Here's how the part is built. I have some questions about the finished solid (model axes, mm). Face numbers are marked on the shaded views. Round coordinates to 2 decimals unless told otherwise and drop trailing zeros. Loops run counter-clockwise (first coordinate to the right, second up) from the corner with the lowest first, then second, coordinate; pieces in that order, holes last. Notation, with made-up numbers: M 10.5,66 L 29.5,66 A26 ccw 29.5,87 Z; hole C 13.5,70.25 d8. An arc over 180 degrees is marked long. Use a Markdown table: item, result.
from build123d import *

# Parameters (mm, degrees)
SKETCH_1_W                   = 20
SKETCH_1_H                   = 50
SKETCH_1_R                   = 3.3
SCREW_BRACKET_20X50X40_DEPTH = 40
SKETCH_2_R                   = 4.25
M10_TAP_PILOT_8P5_DEPTH      = 20


with BuildPart() as part:
    # 草图1 → Screw_bracket_20x50x40 (new body)
    with BuildSketch(Plane.XY):
        with Locations((10, 25)):
            Rectangle(SKETCH_1_W, SKETCH_1_H)
        with Locations((10, 8)):
            Circle(SKETCH_1_R, mode=Mode.SUBTRACT)
        with Locations((10, 42)):
            Circle(SKETCH_1_R, mode=Mode.SUBTRACT)
    extrude(amount=SCREW_BRACKET_20X50X40_DEPTH)

    # 草图2 → M10_tap_pilot_8p5 (cut)
    with BuildSketch(Plane.ZY):
        with Locations((20, 25)):
            Circle(SKETCH_2_R)
    extrude(amount=-M10_TAP_PILOT_8P5_DEPTH, mode=Mode.SUBTRACT)


solid = part.part
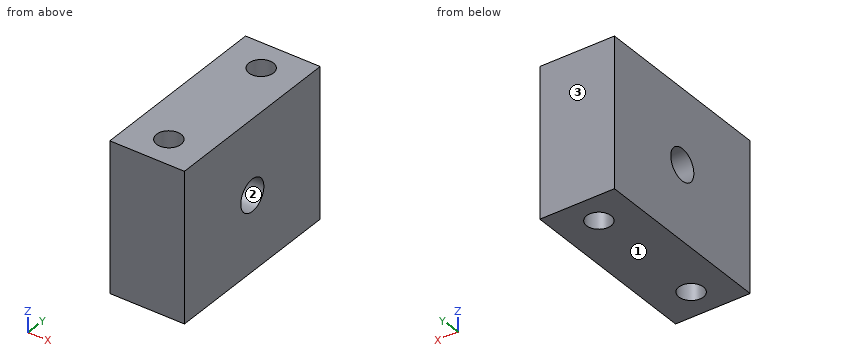
1. Imagine slicing it at D-D, the plane z = 9.5. Write out the boundary of the cut face in (x, y), then the cut area to 3 significant figures.
Answer sheet:
| item | result |
|---|---|
| outline | M 0,0 L 20,0 L 20,50 L 0,50 Z; hole C 10,8 d6.6; hole C 10,42 d6.6 |
| area | 932 mm2 |
2. Imagine slicing it at A-A, the plane z = 18. Write out the boundary of the cut face in (x, y).
Answer sheet:
| item | result |
|---|---|
| outline | M 0,0 L 20,0 L 20,21.25 L 0,21.25 Z; M 0,28.75 L 20,28.75 L 20,50 L 0,50 Z; hole C 10,8 d6.6; hole C 10,42 d6.6 |
3. I need wall thicknesses on probe 1 along Y at (x, z) = (10, 10); probe 2 along Y at (x, z) = (8, 17); probe 3 along Y at (x, z) = (10, 17). Which ranges of each line are inside material? Lowest first, please. Write a range as from..to.
Answer sheet:
| item | result |
|---|---|
| probe 1 | 0..4.7, 11.3..38.7, 45.3..50 |
| probe 2 | 0..5.38, 10.62..21.99, 28.01..39.38, 44.62..50 |
| probe 3 | 0..4.7, 11.3..21.99, 28.01..38.7, 45.3..50 |
4. Imagine slicing it at C-C, the plane y = 42. Write out the boundary of the cut face in (x, z), then the cut area to 3 significant figures.
Answer sheet:
| item | result |
|---|---|
| outline | M 0,0 L 6.7,0 L 6.7,40 L 0,40 Z; M 13.3,0 L 20,0 L 20,40 L 13.3,40 Z |
| area | 536 mm2 |
5. We'd pull the mould along Y, two halves only. Please class the marked faces 1, 2 and 3: +Y half, -Y half, draft (parallel to the pull), parting line (faces both ways), or undercut.
Answer sheet:
| item | result |
|---|---|
| face 1 | draft |
| face 2 | undercut |
| face 3 | +Y half |
6. Imagine slicing it at B-B, the plane x = 10. Write out the boundary of the cut face in (y, z).
Answer sheet:
| item | result |
|---|---|
| outline | M 0,0 L 4.7,0 L 4.7,40 L 0,40 Z; M 11.3,0 L 38.7,0 L 38.7,40 L 11.3,40 Z; M 45.3,0 L 50,0 L 50,40 L 45.3,40 Z; hole C 25,20 d8.5 |
